Here's the drawing with two shaded views (mm, measured from the low corner). I have some questions. A direction names the side the tool comes from. Coordinates: 2 decimals unless noted, no trailing zeros. Write each loop counter-clockwise with the first axis right and the second up, starting at its lowest first coordinate (ties: lowest second). Pieces come first, ordered by that corner, then holes.
Item 1: For P1, Ø2, axis at x = 7, z = 10.5, coming from the +Y side; P2, Ø8, axis at x = 5, z = 18.5, coming from the +Y side; P3, Ø1.5, axis at x = 9.5, y = 18.5, coming from the -Z side (1 decimal), each with a flat end and sliding along its axis, tell me the tip position at first contact or that it passes through.
Item 2: I want a section at A-A on y = 11.75. Please give me the cut outline in (x, z) (1 decimal), then the cut area to 3 significant figures.
Item 3: Thinking about a two-plate mould opening in Y: for the marked faces 1, 2 and 3, which applies, +Y half, -Y half, draft (parallel to the pull), parting line (faces both ways), or undercut?
Item 4: I want a section at B-B on x = 6.25. Please give me the cut outline in (y, z) (1 decimal).
Item 5: Which directions (+Z, -Z, +X, -X, +Y, -Y) give clear straight access to the entire face, cutting with the end or side of a thin tool? Please do the marked faces 4 and 5.
Item 6: I want a section at C-C on y = 16.25. Please give me the cut outline in (x, z) (1 decimal), then the cut area to 3 significant figures.
Item 7: If I drill on probe 1 along Y at (x, z) = (11, 13.75) (1 decimal); probe 2 along Z at (x, y) = (18.25, 11.5) (1 decimal), over which ranges is the centre line in solid material (lowest first)?
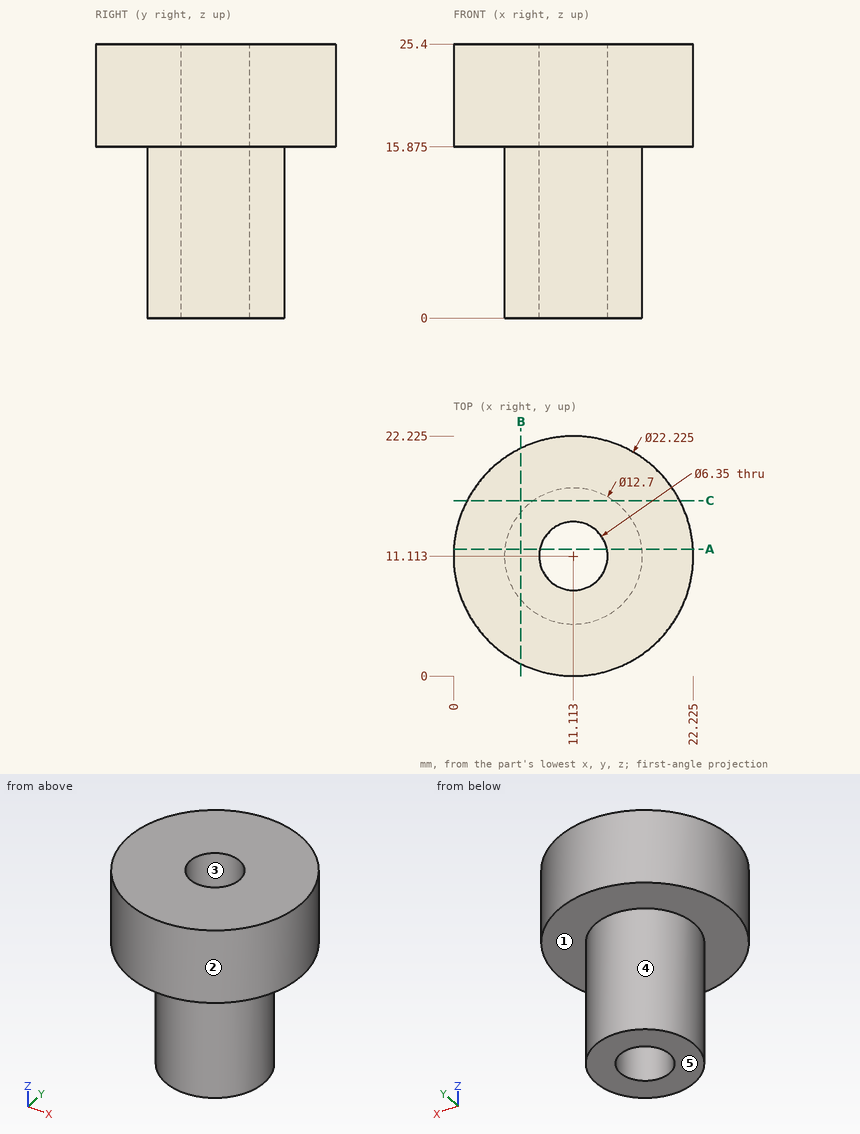
Response values:
1. P1: stops at y = 16.65
1. P2: stops at y = 22.02
1. P3: stops at z = 15.9
2. outline: (0, 15.9) - (4.8, 15.9) - (4.8, 0) - (8, 0) - (8, 25.4) - (0, 25.4) - close; (14.2, 0) - (17.4, 0) - (17.4, 15.9) - (22.2, 15.9) - (22.2, 25.4) - (14.2, 25.4) - close
2. area: 254 mm2
3. face 1: draft
3. face 2: parting line
3. face 3: undercut
4. outline: (1.1, 15.9) - (7, 15.9) - (7, 0) - (15.2, 0) - (15.2, 15.9) - (21.1, 15.9) - (21.1, 25.4) - (1.1, 25.4) - close
5. face 4: -Z
5. face 5: -Z, +X, -X, +Y, -Y
6. outline: (1.3, 15.9) - (7.4, 15.9) - (7.4, 0) - (14.8, 0) - (14.8, 15.9) - (21, 15.9) - (21, 25.4) - (1.3, 25.4) - close
6. area: 306 mm2
7. probe 1: y = 4.8 to 7.9, 14.3 to 17.5
7. probe 2: z = 15.9 to 25.4
